Can you work these out from the model? Positions are in its coordinate system, mm. A direction names the side the tool comes from. Coordinates: 2 decimals unless noted, no trailing zeros. Order: outer loops, then holes, each group sorted by start corner. A loop starts at its lowest first (then second) coordinate and runs counter-clockwise, first axis right, second up. Notation, with made-up numbers: (2.5, -4) -> (7.5, -4) arc R20 ccw to (7.5, 19) -> close; hole circle Ø3 at (24.25, 37.5). An arc over 180 degrees is marked (long way). Answer as a JSON object with one key per item and string values. Group by question number.
(1) I want a section at D-D, the plane x = 16. List the corners of the cut face in (y, z) for me.
(2) I want a section at B-B, the plane y = 0. List the corners of the cut face in (x, z) for me.
(3) I want a section at A-A, the plane x = 0. List the corners of the cut face in (y, z) for me, plus the area to 3 significant figures.
(4) For pin 1 (2.5 mm diameter, centred on x = -5.75, y = 9.96, fed in from +Z); pin 2 (1 mm diameter, centred on x = -17, y = -10.5, fed in from -Z); pin 3 (3.5 mm diameter, centred on x = 11.5, y = 0, fed in from +Z); pin 4 (6 mm diameter, centred on x = -17.5, y = -11.5, fed in from +Z), each with a flat end and sliding along its axis, tell me the tip position at first contact or that it passes through.
(5) If we mould it in two halves opening along Y, with no side actions, what happens to faces 1 (the cylindrical face through (13.887, 10.648, -0.493)), 2 (the cylindrical face through (-6.86, -8.95, 15.22)), 3 (the flat face through (-17, -5, 0))? For each: pulls with the +Y half, pulls with the -Y half, needs draft (parallel to the pull), parting line crosses it, or undercut.
(6) Which directions (+Z, -Z, +X, -X, +Y, -Y) give clear straight access to the entire face, cutting with the end or side of a thin tool? Please do faces 4 (the flat face through (-17, -5, 30)), 5 (the cylindrical face through (-6, 0, 15)).
(7) I need wall thicknesses on line 1 (Y direction, x = 0, z = 13); line 2 (Y direction, x = -7, z = 2); line 3 (Z direction, x = 17, y = -13). Which ranges of each line are inside material? Lowest first, please.
(8) I want a section at C-C, the plane z = 18.5. List the corners of the cut face in (x, y) for me, plus the area to 3 significant figures.
Autodesk Inventor part; units mm, degrees
ref_plane "YZ Plane" through (0, 0, 0) normal (1, 0, 0) x (0, 1, 0)
ref_plane "XZ Plane" through (0, 0, 0) normal (0, 1, 0) x (-1, 0, 0)
ref_plane "XY Plane" through (0, 0, 0) normal (0, 0, 1) x (1, 0, 0)
sketch "Skizze1" plane through (0, 0, 0) normal (0, 0, 1) x (1, 0, 0)
  circle A0 centre (0, 0) radius 17.5
  dimension "d1" = 35
extrude "Extrusion1" add sketch "Skizze1" along normal blind 31
sketch "Skizze2" plane through (0, 0, 0) normal (0, 0, -1) x (-1, 0, 0)
  point P0 (0, 0)
ref_plane "Arbeitsebene1" through (0, 0, 0) normal (0, 0, 1) x (1, 0, 0)
sketch "Skizze3" plane through (0, 0, 0) normal (0, 0, 1) x (1, 0, 0)
  circle A0 centre (0, 0) radius 25
  dimension "d7" = 50
extrude "Extrusion3" add sketch "Skizze3" along normal blind 30
sketch "Skizze4" plane through (0, 0, 0) normal (0, 0, -1) x (-1, 0, 0)
  circle A0 centre (0, 0) radius 17.5
extrude "Extrusion4" add sketch "Skizze4" along normal blind 1
sketch "Skizze5" plane through (0, 0, 31) normal (0, 0, 1) x (1, 0, 0)
  line L0 (0, 0) -> (11.5, 0) construction
  line L1 (0, 0) -> (11.5, 0) construction
  circle A0 centre (-5.75, -9.9593) radius 1.5
  circle A1 centre (-5.75, 9.9593) radius 1.5
  circle A2 centre (11.5, 0) radius 1.5
  circle A3 centre (0, 0) radius 6
  dimension "d18" = 3
  dimension "d19" = 3
  dimension "d20" = 3
  dimension "d21" = 12
extrude "Extrusion5" cut sketch "Skizze5" against normal through all
properties part number "Drohnenrad"
Computed values:
{
 "1": {"outline": "(-19.21, 0) -> (-7.09, 0) -> (-7.09, -1) -> (7.09, -1) -> (7.09, 0) -> (19.21, 0) -> (19.21, 30) -> (7.09, 30) -> (7.09, 31) -> (-7.09, 31) -> (-7.09, 30) -> (-19.21, 30) -> close"},
 "2": {"outline": "(-25, 0) -> (-17.5, 0) -> (-17.5, -1) -> (-6, -1) -> (-6, 31) -> (-17.5, 31) -> (-17.5, 30) -> (-25, 30) -> close; (6, -1) -> (10, -1) -> (10, 31) -> (6, 31) -> close; (13, -1) -> (17.5, -1) -> (17.5, 0) -> (25, 0) -> (25, 30) -> (17.5, 30) -> (17.5, 31) -> (13, 31) -> close"},
 "3": {"outline": "(-25, 0) -> (-17.5, 0) -> (-17.5, -1) -> (-6, -1) -> (-6, 31) -> (-17.5, 31) -> (-17.5, 30) -> (-25, 30) -> close; (6, -1) -> (17.5, -1) -> (17.5, 0) -> (25, 0) -> (25, 30) -> (17.5, 30) -> (17.5, 31) -> (6, 31) -> close", "area": "1,190 mm2"},
 "4": {"pin 1": "passes through", "pin 2": "stops at z = 0", "pin 3": "stops at z = 31", "pin 4": "stops at z = 30"},
 "5": {"face 1": "parting line crosses it", "face 2": "undercut", "face 3": "needs draft"},
 "6": {"face 4": "+Z", "face 5": "+Z, -Z"},
 "7": {"line 1": "y = -25 to -6, 6 to 25", "line 2": "y = -24 to -10.79, -9.13 to 9.13, 10.79 to 24", "line 3": "z = 0 to 30"},
 "8": {"outline": "circle Ø50 at (0, 0); hole circle Ø3 at (-5.75, -9.96); hole circle Ø3 at (-5.75, 9.96); hole circle Ø12 at (0, 0); hole circle Ø3 at (11.5, 0)", "area": "1,830 mm2"}
}
